Input: part model. Units: mm. Frame: model coordinates. A direction names the side the tool comes from. Coordinates: 2 decimals unless noted, no trailing zeros. Write each loop counter-clockwise with the first axis right and the second up, starting at its lowest first coordinate (ties: lowest second). Pieces come first, ordered by that corner, then holes.
1) Draft query along Y for faces 1 (the flat face through (112, 0, 0)), 2 (the cylindrical face through (54.23, 3.755, -11.923)), 3 (the cylindrical face through (54.23, -13.18, 2.93)). Return one class per face: pulls with the +Y half, pulls with the -Y half, needs draft (parallel to the pull), parting line crosses it, or undercut.
2) Line query: L1, parallel to Y at x = 63, z = 0; L2, parallel to X at y = 9, z = 0.25; L3, parallel to Z at x = 17, y = 9. Output: solid intervals per line, ascending.
3) Section query C-C (x = 8.5). Output: boundary loops of the cut face in (y, z), then the cut area to 3 significant figures.
4) Pin query (flat end, axial travel): pin 1 Ø4 at (x, y) = (64.5, -8) entering from -Z; pin 2 Ø8 at (x, z) = (45, -1.5) entering from -Y; pin 3 Ø1.5 at (x, z) = (56.5, -7.5) entering from -Y. Return the tip coordinate at first contact, or that it passes through.
5) Set-up query: faces 4 (the flat face through (0, -9, -9)), 5 (the flat face through (110, 0, 0)). Return all of +Z, -Z, +X, -X, +Y, -Y with unobstructed straight access to the full face (end or side cutting, diameter ignored); none if empty.
from build123d import *

# Parameters (mm, degrees)
SKETCH1_R           = 13.5
SKETCH1_R_2         = 12.5
BOSS_EXTRUDE5_DEPTH = 110
SKETCH4_R           = 15
BOSS_EXTRUDE6_DEPTH = 2
FILLET7_R           = 1


with BuildPart() as part:
    # Sketch1 → Boss-Extrude5 (new body)
    with BuildSketch(Plane(origin=(0, 0, 0), x_dir=(0, 0, -1), z_dir=(1, 0, 0))):
        Circle(SKETCH1_R)
        Circle(SKETCH1_R_2, mode=Mode.SUBTRACT)
    extrude(amount=BOSS_EXTRUDE5_DEPTH)

    # Sketch4 → Boss-Extrude6 (add)
    with BuildSketch(Plane(origin=(110, 0, 0), x_dir=(0, 0, -1), z_dir=(1, 0, 0))):
        Circle(SKETCH4_R)
    extrude(amount=BOSS_EXTRUDE6_DEPTH)

    # Fillet7
    fillet7_edges = [part.edges().sort_by_distance(p)[0] for p in [
        (110, 0, 15),
        (112, 0, 15),
    ]]
    fillet(fillet7_edges, radius=FILLET7_R - 0.0001)  # a hair under: the kernel refuses the full size


solid = part.part
Answer:
1. face 1: needs draft
1. face 2: undercut
1. face 3: parting line crosses it
2. L1: y = -13.5 to -12.5, 12.5 to 13.5
2. L2: x = 110 to 112
2. L3: z = -10.06 to -8.67, 8.67 to 10.06
3. outline: circle Ø27 at (0, 0); hole circle Ø25 at (0, 0)
3. area: 81.7 mm2
4. pin 1: stops at z = -12.09
4. pin 2: stops at y = -13.5
4. pin 3: stops at y = -11.69
5. face 4: +Z, -Z, -X, +Y, -Y
5. face 5: -X
